Here's how the part is built. I have some questions about the finished solid (model axes, mm). A direction names the side the tool comes from. Give positions to 0.01 mm unless a question says otherwise; leave off trailing zeros. Loops run counter-clockwise (first coordinate to the right, second up) from the corner with the lowest first, then second, coordinate; pieces in that order, holes last.
Q1. Will these pins go through, and if not, where does the flat tip stop? P1, Ø2, axis at x = 17, z = -19, coming from the -Y side; P2, Ø5, axis at y = -45.5, z = 8, coming from the +X side; P3, Ø10.5, axis at x = 0, z = 25, coming from the +Y side; P4, Ø2, axis at x = 9.5, y = -17.5, coming from the -Z side.
Q2. For faces 4 (the face through (-14, 0, 14)), 5 (the face through (0.143, 3.042, 21.753)), 6 (the face through (-11.8, 3.7, 10.3)), which set-ups out of +Z, -Z, +X, -X, +Y, -Y let a thin tool reach every point of the face, with its end or its side?
Q3. If we section it at B-B (y = -37.5): Please give me the cut outline in (x, z).
Q4. I need wall thicknesses on line 1 (X direction, y = 4, z = 0); line 2 (X direction, y = 1.35, z = 0); line 3 (Y direction, x = 17, z = -20). Which ranges of each line are inside material? Lowest first, please.
Q5. We'd pull the mould along X, two halves only. Please class faces 1 (the face through (0.143, 3.042, -28.247)), 2 (the face through (-31.24, 2.96, -6.94)), 3 (the face through (0, 6, 21)): +X half, -X half, draft (parallel to the pull), parting line (faces both ways), or undercut.
Q6. If we section it at A-A (z = 0): Give the number of separate pieces and of enclosed holes in the cut face, plus the area to 4 significant figures.
from build123d import *

# Parameters (mm, degrees)
SKETCH1_R           = 32
BOSS_EXTRUDE1_DEPTH = 6
SKETCH2_R           = 17.5
BOSS_EXTRUDE2_DEPTH = 54
SKETCH3_R           = 20
CUT_EXTRUDE1_DEPTH  = 2.3
SKETCH4_R           = 15
CUT_EXTRUDE2_DEPTH  = 74.3300075
SKETCH5_R           = 3.25
CUT_EXTRUDE3_DEPTH  = 76.153176912
CHAMFER1_SIZE       = 0.5


with BuildPart() as part:
    # Sketch1 → Boss-Extrude1 (new body)
    with BuildSketch(Plane(origin=(0, 0, 0), x_dir=(1, 0, 0), z_dir=(0, 1, 0))):
        with Locations(Location((0, 0, 0), (0, 0, 270))):
            Circle(SKETCH1_R)
    extrude(amount=BOSS_EXTRUDE1_DEPTH)

    # Sketch2 → Boss-Extrude2 (add)
    with BuildSketch(Plane.XZ):
        with Locations(Location((0, 0, 0), (0, 0, 270))):
            Circle(SKETCH2_R)
    extrude(amount=BOSS_EXTRUDE2_DEPTH)

    # Sketch3 → Cut-Extrude1 (cut)
    with BuildSketch(Plane(origin=(0, 6, 0), x_dir=(1, 0, 0), z_dir=(0, 1, 0))):
        with Locations(Location((0, 0, 0), (0, 0, 270))):
            Circle(SKETCH3_R)
    extrude(amount=-CUT_EXTRUDE1_DEPTH, mode=Mode.SUBTRACT)

    # Sketch4 → Cut-Extrude2 (cut, through all)
    with BuildSketch(Plane(origin=(0, 3.7, 0), x_dir=(1, 0, 0), z_dir=(0, 1, 0))):
        with Locations(Location((0, 0, 0), (0, 0, 270))):
            Circle(SKETCH4_R)
    extrude(amount=-CUT_EXTRUDE2_DEPTH, mode=Mode.SUBTRACT)

    # Sketch5 → Cut-Extrude3 (cut, through all)
    with BuildSketch(Plane(origin=(0, 6, 0), x_dir=(1, 0, 0), z_dir=(0, 1, 0))):
        with Locations(Location((0, 25, 0), (0, 0, 270))):
            Circle(SKETCH5_R)
        with Locations(Location((25, 0, 0), (0, 0, 270))):
            Circle(SKETCH5_R)
        with Locations(Location((0, -25, 0), (0, 0, 270))):
            Circle(SKETCH5_R)
        with Locations(Location((-25, 0, 0), (0, 0, 270))):
            Circle(SKETCH5_R)
    extrude(amount=-CUT_EXTRUDE3_DEPTH, mode=Mode.SUBTRACT)

    # Chamfer1
    chamfer1_edges = [part.edges().sort_by_distance(p)[0] for p in [
        (0, 6, -20),
        (0, -54, -15),
        (0, 3.7, -15),
        (0, 0, -32),
        (0, 6, -32),
        (0, -54, 17.5),
    ]]
    chamfer(chamfer1_edges, length=CHAMFER1_SIZE)


solid = part.part
Check sheet entries:
1. P1: stops at y = 0
1. P2: stops at x = 16.61
1. P3: stops at y = 6
1. P4: stops at z = -15.3
2. face 4: -Y
2. face 5: +Y, -Y
2. face 6: +Y
3. outline: circle Ø35 at (0, 0); hole circle Ø30 at (0, 0)
4. line 1: x = -32 to -28.25, -21.75 to -20, 20 to 21.75, 28.25 to 32
4. line 2: x = -32 to -28.25, -21.75 to -15, 15 to 21.75, 28.25 to 32
4. line 3: y = 0 to 6
5. face 1: undercut
5. face 2: parting line
5. face 3: draft
6. separate pieces: 4
6. enclosed holes: 0
6. area: 371.5 mm2
